from build123d import *

# Parameters (mm, degrees)
F0_W     = 276.225
F0_H     = 150.9410084384
F1_DEPTH = 25.4
F3_DEPTH = 25.4


with BuildPart() as f1:
    # F0 (on Front) → F1 (new body)
    with BuildSketch(Plane.XZ):
        Rectangle(F0_W, F0_H)
    extrude(amount=F1_DEPTH)

    # F2 (on face) → F3 (cut)
    with BuildSketch(Plane.XZ.offset(25.4)):
        Polygon((-138.1125, 15.167717062), (-24.4453392207, 75.4705042192), (-138.1125, 75.4705042192), align=None)
        Polygon((-138.1125, -75.4705042192), (-24.4453392207, -75.4705042192), (-138.1125, -15.167717062), align=None)
        Polygon((138.1125, 75.4705042192), (26.3546607793, 75.4705042192), (138.1125, 16.1806517634), align=None)
        Polygon((138.1125, -16.1806517634), (26.3546607793, -75.4705042192), (138.1125, -75.4705042192), align=None)
        with BuildLine():
            Line((0.9546607793, -32.84869415), (0.9546607793, 33.82630585))
            ThreePointArc((0.9546607793, 33.82630585), (0.6912380103, 33.8252650905), (0.4278316888, 33.822142877))
            ThreePointArc((0.4278316888, 33.822142877), (-32.3817984612, 0.225383081), (0.9546607793, -32.84869415))
        make_face()
        with BuildLine():
            ThreePointArc((0.9546607793, -32.84869415), (24.5278330971, -23.0843664678), (34.2921607793, 0.48880585))
            ThreePointArc((34.2921607793, 0.48880585), (24.5278330971, 24.0619781678), (0.9546607793, 33.82630585))
            Line((0.9546607793, 33.82630585), (0.9546607793, -32.84869415))
        make_face()
        with BuildLine():
            Line((-131.7264735699, -10.232282938), (-42.1830345138, -10.232282938))
            ThreePointArc((-42.1830345138, -10.232282938), (-43.4473379757, 2.5539950823), (-41.0016506128, 15.167717062))
            Line((-41.0016506128, 15.167717062), (-131.7264735699, 15.167717062))
            Line((-131.7264735699, 15.167717062), (-131.7264735699, -10.232282938))
        make_face()
        with BuildLine():
            Line((130.1703900099, 15.167717062), (42.9109721714, 15.167717062))
            ThreePointArc((42.9109721714, 15.167717062), (44.7768043906, 7.9334166062), (45.4046607793, 0.48880585))
            ThreePointArc((45.4046607793, 0.48880585), (45.0753648522, -4.9117470949), (44.0923560724, -10.232282938))
            Line((44.0923560724, -10.232282938), (130.1703900099, -10.232282938))
            Line((130.1703900099, -10.232282938), (130.1703900099, 15.167717062))
        make_face()
    extrude(amount=-F3_DEPTH, mode=Mode.SUBTRACT)


solid = f1.part
Can you work these out from the model? Positions are in its coordinate system, mm. A direction names the side the tool comes from. Give positions to 0.01 mm unless a question says otherwise; leave off trailing zeros. Order: outer loops, then holes, each group sorted by start corner. A loop starts at its lowest first (then second) coordinate and runs counter-clockwise, first axis right, second up. Notation, with made-up numbers: M 33.5,48.5 L 85.5,48.5 A24 ccw 85.5,78.5 Z; hole C -31.75,-30 d1. An arc over 180 degrees is marked long. Use one line per item in the form item = value.
Item 1: Will these pins go through, and if not, where does the flat tip stop? pin 1 Ø8 at (x, z) = (71, -41.5) entering from +Y; pin 2 Ø12.5 at (x, y) = (-95.5, -15.5) entering from +Z; pin 3 Ø8 at (x, y) = (105, -17) entering from +Z; pin 4 Ø10 at (x, z) = (103.5, -5) entering from -Y.
Values follow:
pin_1 = 0
pin_2 = 41.09
pin_3 = 35.87
pin_4 = through
Item 2: If I drill on line 1 along X through (y, z) = (-18.5, -1.5); line 2 along X through (y, z) = (-22, -2); line 3 along Z through (x, y) = (24.5, -14.75), over which ranges is the centre line in solid material (lowest first)? Write a range as [from, to].
Values follow:
line_1 = [-138.11, -131.73], [-43.45, -32.32], [34.23, 45.36], [130.17, 138.11]
line_2 = [-138.11, -131.73], [-43.43, -32.29], [34.2, 45.33], [130.17, 138.11]
line_3 = [-75.47, -23.11], [24.09, 75.47]
Item 3: For faces 4 (the flat face through (87, -13, 15.168)), 5 (the flat face through (-33, -25.4, 1)), which set-ups out of +Z, -Z, +X, -X, +Y, -Y let a thin tool reach every point of the face, with its end or its side?
Values follow:
face_4 = +Y, -Y
face_5 = +Z, -Z, +X, -X, -Y
Item 4: If we section it at C-C, the plane z = 7: Write out the boundary of the cut face in (x, y), and give its area (3 significant figures).
Values follow:
outline = M -138.11,-25.4 L -131.73,-25.4 L -131.73,0 L -138.11,0 Z; M -43.02,-25.4 L -31.74,-25.4 L -31.74,0 L -43.02,0 Z; M 33.65,-25.4 L 44.93,-25.4 L 44.93,0 L 33.65,0 Z; M 130.17,-25.4 L 138.11,-25.4 L 138.11,0 L 130.17,0 Z
area = 937 mm^2
Item 5: If we section it at B-B, the plane x = -101: Write out the boundary of the cut face in (y, z).
Values follow:
outline = M -25.4,-34.86 L 0,-34.86 L 0,-10.23 L -25.4,-10.23 Z; M -25.4,15.17 L 0,15.17 L 0,34.86 L -25.4,34.86 Z
Item 6: Thinking about a two-plate mould opening in Z: for faces 1 (the flat face through (87, -13, -10.232)), 2 (the flat face through (-80.483, -12.878, -45.741)), 3 (the flat face through (81.45, -12.88, 46.24)), which applies, pulls with the +Z half, pulls with the -Z half, needs draft (parallel to the pull), parting line crosses it, or undercut?
Values follow:
face_1 = undercut
face_2 = pulls with the -Z half
face_3 = pulls with the +Z half
Item 7: If we section it at D-D, the plane z = 26: Write out the boundary of the cut face in (x, y).
Values follow:
outline = M -117.69,-25.4 L -20.51,-25.4 L -20.51,0 L -117.69,0 Z; M 22.42,-25.4 L 119.6,-25.4 L 119.6,0 L 22.42,0 Z
Item 8: If we section it at A-A, the plane y = -6: Count the separate pieces of the cut face and the enclosed holes in it, and give its area (3 significant figures).
Values follow:
separate_pieces = 1
enclosed_holes = 3
area = 20,300 mm^2
